```python
from build123d import *

# Parameters (mm, degrees)
ESQUISSE1_R             = 7.15
ESQUISSE1_R_2           = 3.15
BOSS_EXTRU_1_DEPTH      = 5
BOSS_EXTRU_2_DEPTH      = 5
BOSS_EXTRU_3_START      = -2
ESQUISSE3_R             = 3.15
ESQUISSE3_R_2           = 1.5
BOSS_EXTRU_3_DEPTH      = 2
BOSS_EXTRU_5_DEPTH      = 10
ENL_V_MAT_EXTRU_1_DEPTH = 5


with BuildPart() as part:
    # Esquisse1 → Boss.-Extru.1 (new body)
    with BuildSketch(Plane.XY):
        Circle(ESQUISSE1_R)
        Circle(ESQUISSE1_R_2, mode=Mode.SUBTRACT)
    extrude(amount=BOSS_EXTRU_1_DEPTH)

    # Esquisse2 → Boss.-Extru.2 (add)
    with BuildSketch(Plane.XY.offset(5)):
        with BuildLine():
            Line((-0.926838299, 7.08967353), (6.743880262, 2.375411335))
            add(Edge.make_bspline(
                [(34.021054956, -0.824268448), (15.778325112, 19.117081856), (6.743880262, 2.375411335)],
                knots=[0, 0, 0, 1, 1, 1], degree=2))
            add(Edge.make_bspline(
                [(35.905224024, 0.760247249), (37.183183912, -2.67189548), (34.021054956, -0.824268448)],
                knots=[0, 0, 0, 1, 1, 1], degree=2))
            add(Edge.make_bspline(
                [(-0.926838299, 7.08967353), (15.737638427, 28.114370549), (35.905224024, 0.760247249)],
                knots=[0, 0, 0, 1, 1, 1], degree=2))
        make_face()
    extrude(amount=-BOSS_EXTRU_2_DEPTH)

    # Esquisse3 → Boss.-Extru.3 (add)
    with BuildSketch(Plane.XY.offset(5).offset(BOSS_EXTRU_3_START)):
        Circle(ESQUISSE3_R)
        Circle(ESQUISSE3_R_2, mode=Mode.SUBTRACT)
    extrude(amount=BOSS_EXTRU_3_DEPTH)

    # Esquisse6 → Boss.-Extru.5 (add)
    with BuildSketch(Plane.XY.offset(5)):
        with BuildLine():
            Line((37.162166163, 2.495785683), (41.863791518, -2.205839672))
            ThreePointArc((41.863791518, -2.205839672), (42.156684737, -2.912946454), (41.863791518, -3.620053235))
            Line((41.863791518, -3.620053235), (38.837480033, -6.646364721))
            ThreePointArc((38.837480033, -6.646364721), (38.148081452, -6.939101137), (37.448749191, -6.670960502))
            Line((37.448749191, -6.670960502), (32.580530811, -2.135928171))
            ThreePointArc((32.580530811, -2.135928171), (32.262311674, -1.421933809), (32.55504809, -0.697118827))
            add(Edge.make_bspline(
                [(32.55504809, -0.697118827), (33.011349081, 1.483281056), (31.368103593, 3.24060207)],
                knots=[0, 0, 0, 1, 1, 1], degree=2))
            Line((31.368103593, 3.24060207), (32.92139501, 4.017247779))
            add(Edge.make_bspline(
                [(35.7479526, 2.495785683), (33.974850615, 2.525051405), (32.92139501, 4.017247779)],
                knots=[0, 0, 0, 1, 1, 1], degree=2))
            ThreePointArc((35.7479526, 2.495785683), (36.455059382, 2.788678902), (37.162166163, 2.495785683))
        make_face()
    extrude(amount=-BOSS_EXTRU_5_DEPTH)

    # Esquisse7 → Enlèv. mat.-Extru.1 (cut)
    with BuildSketch(Plane(origin=(0, 0, -5), x_dir=(-1, 0, 0), z_dir=(0, 0, -1))):
        Polygon((-35.7479526, 2.495785683), (-32.55504809, -0.697118827), (-29.617226271, 2.240702992), (-34.427657246, 5.5904913), align=None)
    extrude(amount=-ENL_V_MAT_EXTRU_1_DEPTH, mode=Mode.SUBTRACT)


solid = part.part
```
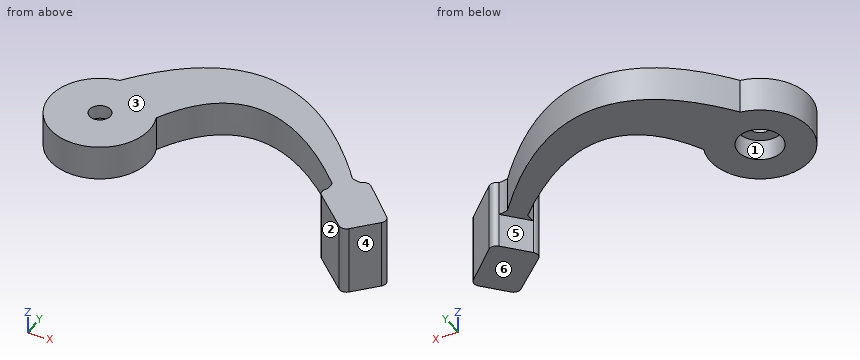
Part model, mm, in its own coordinate system. Face numbers are marked on the shaded views. A direction names the side the tool comes from. Give positions to 0.01 mm unless a question says otherwise; leave off trailing zeros. Use a Markdown table: item, result. Add a question column.
(1) Mould opens along X. For the marked faces 1, 2, 3 and 4 say: +X half, -X half, draft (parallel to the pull), parting line (faces both ways), or undercut.
(2) Drop flat-ended pins along their axis: P1, Ø4, axis at x = 10, z = 3.5, coming from the -Y side; P2, Ø1.5, axis at x = 3, z = 2, coming from the +Y side; P3, Ø2.5, axis at x = 0, y = 0, coming from the -Z side (3 decimals); P4, Ø3, axis at y = -4.5, z = 2, coming from the -X side. Give the stop position or say it passes through.
(3) 3-axis set-ups, long thin cutter, end or side, ignore diameter. For the marked faces 5 and 6: which of +Z, -Z, +X, -X, +Y, -Y reach the whole face in a straight line?
(4) Probe line 1 along Z through (x, y) = (5, -5); line 2 along Y through (x, z) = (0, 3.75); line 3 along Y through (x, z) = (0, 1.3). List the from-to ranges inside material, lowest first. Write a range as [from, to].
(5) Saw through at A-A, the plane y = 0. Give the number of separate pieces and of enclosed holes in the cut face, and give its area (3 significant figures).
Answer key:
| question | item | result |
|---|---|---|
| 1 | face 1 | undercut |
| 1 | face 2 | undercut |
| 1 | face 3 | draft |
| 1 | face 4 | +X half |
| 2 | P1 | y = 4.46 |
| 2 | P2 | y = 11.98 |
| 2 | P3 | through |
| 2 | P4 | x = -6.49 |
| 3 | face 5 | -Z, -X, +Y |
| 3 | face 6 | -Z, +X, -X, +Y, -Y |
| 4 | line 1 | [0, 5] |
| 4 | line 2 | [-7.15, -1.5], [1.5, 8.22] |
| 4 | line 3 | [-7.15, -3.15], [3.15, 8.22] |
| 5 | separate pieces | 3 |
| 5 | enclosed holes | 0 |
| 5 | area | 114 mm^2 |
